```python
from build123d import *

# Parameters (mm, degrees)
SKETCH1_W                = 100
SKETCH1_H                = 110
BOSS_EXTRUDE1_DEPTH      = 6.86
BOSS_EXTRUDE2_DEPTH      = 6.86
CUT_EXTRUDE1_DEPTH       = 84.419927529
CUT_EXTRUDE1_DEPTH_BACK  = 84.419927529
CUT_EXTRUDE5_DEPTH       = 84.419927529
CUT_EXTRUDE6_DEPTH       = 84.419927529
SKETCH7_W                = 42
SKETCH7_H                = 3.55
CUT_EXTRUDE7_DEPTH       = 84.419927529
SKETCH8_W                = 5
SKETCH8_H                = 7.62
CUT_EXTRUDE8_DEPTH       = 84.419927529
CUT_EXTRUDE9_DEPTH       = 84.419927529
LPATTERN1_COUNT          = 2
LPATTERN1_PITCH          = 49.4
SKETCH15_W               = 6.5
SKETCH15_H               = 9.5
BOSS_EXTRUDE3_DEPTH      = 6.86
CUT_EXTRUDE14_START      = -6.86
CUT_EXTRUDE14_DEPTH      = 6.86
BOSS_EXTRUDE4_DEPTH      = 6.86
FILLET3_R                = 5
FILLET4_R                = 7
CUT_EXTRUDE11_DEPTH      = 84.419927529
BOSS_EXTRUDE5_DEPTH      = 6.86
CUT_EXTRUDE12_DEPTH      = 84.419927529
CUT_EXTRUDE12_DEPTH_BACK = 84.419927529
SKETCH21_R               = 1
CUT_EXTRUDE13_DEPTH      = 84.419927529
CUT_EXTRUDE15_DEPTH      = 84.419927529
CUT_EXTRUDE15_DEPTH_BACK = 84.419927529
CUT_EXTRUDE16_DEPTH      = 84.419927529
CUT_EXTRUDE16_DEPTH_BACK = 84.419927529
FILLET2_R                = 1
BOSS_EXTRUDE6_DEPTH      = 6.86
CUT_EXTRUDE17_DEPTH      = 84.419927529
BOSS_EXTRUDE9_DEPTH      = 6.86


# Read off the part's stored shape, not the designer's step: Cut-Extrude14
with BuildPart() as part:
    # Sketch1 → Boss-Extrude1 (new body)
    with BuildSketch(Plane.XY):
        Rectangle(SKETCH1_W, SKETCH1_H)
    extrude(amount=BOSS_EXTRUDE1_DEPTH)

    # Sketch14 → Boss-Extrude2 (add)
    with BuildSketch(Plane.XY.offset(6.86)):
        with BuildLine():
            Line((-50, 44), (-56.9, 44))
            Line((-56.9, 44), (-57.252653961, 46))
            Line((-57.252653961, 46), (-60.252653961, 46))
            ThreePointArc((-60.252653961, 46), (-62.140394827, 27.177051725), (-56.9, 9))
            Line((-56.9, 9), (-50, 9))
            Line((-50, 9), (-50, 44))
        make_face()
    extrude(amount=-BOSS_EXTRUDE2_DEPTH)

    # Sketch9 → Cut-Extrude1 (cut, two sides: drawn at the far end of the back side and taken through both)
    with BuildSketch(Plane.XY.offset(6.86).offset(-CUT_EXTRUDE1_DEPTH_BACK)):
        Polygon((-202.691345573, 326.397371639), (-46, 55), (2.5, -29.004464167), (-49.825975731, -59.214880341), (-321.22334737, -215.906225914), (291.08659924, -349.739606366), (409.618601037, 192.563991188), align=None)
    extrude(amount=CUT_EXTRUDE1_DEPTH + CUT_EXTRUDE1_DEPTH_BACK, mode=Mode.SUBTRACT)

    # Sketch11 → Cut-Extrude5 (cut, through all)
    with BuildSketch(Plane.XY.offset(6.86)):
        Polygon((-35.90593882, 37.516573181), (-8.20593882, -10.461234188), (-15.13414205, -14.461234188), (-42.83414205, 33.516573181), align=None)
    extrude(amount=-CUT_EXTRUDE5_DEPTH, mode=Mode.SUBTRACT)

    # Sketch12 → Cut-Extrude6 (cut, through all)
    with BuildSketch(Plane.XY.offset(6.86)):
        Polygon((-18.88414205, -7.96604366), (-21.534179786, -9.49604366), (-35.534179786, 14.752667646), (-32.88414205, 16.282667646), align=None)
    extrude(amount=-CUT_EXTRUDE6_DEPTH, mode=Mode.SUBTRACT)

    # Sketch7 → Cut-Extrude7 (cut, through all)
    with BuildSketch(Plane.XY.offset(6.86)):
        with Locations((-50, -34)):
            Rectangle(SKETCH7_W, SKETCH7_H)
    extrude(amount=-CUT_EXTRUDE7_DEPTH, mode=Mode.SUBTRACT)

    # Sketch8 → Cut-Extrude8 (cut, through all)
    with BuildSketch(Plane.XY.offset(6.86)):
        with Locations((-36.5, -34)):
            Rectangle(SKETCH8_W, SKETCH8_H)
    extrude(amount=-CUT_EXTRUDE8_DEPTH, mode=Mode.SUBTRACT)

    # Sketch13 → Cut-Extrude9 (cut, through all)
    with BuildSketch(Plane.XY.offset(6.86)):
        Polygon((-41.88414205, 31.871124914), (-40.78414205, 29.965869026), (-48.578370684, 25.465869026), (-48.078370684, 24.599843622), (-49.508178626, 23.774343622), (-50.008178626, 24.640369026), (-52.908497703, 22.965869026), (-54.008497703, 24.871124914), (-51.108178626, 26.545624914), (-51.608178626, 27.411650318), (-50.178370684, 28.237150318), (-49.678370684, 27.371124914), align=None)
        Polygon((-39.45593882, 43.665353548), (-38.35593882, 41.76009766), (-46.150167454, 37.26009766), (-45.650167454, 36.394072256), (-47.079975396, 35.568572256), (-47.579975396, 36.43459766), (-50.480294473, 34.76009766), (-51.580294473, 36.665353548), (-48.679975396, 38.339853548), (-49.179975396, 39.205878952), (-47.750167454, 40.031378952), (-47.250167454, 39.165353548), align=None)
        Polygon((-18.443009001, -24.930108514), (-11.443009001, -37.054464167), (-9.537753113, -35.954464167), (-16.537753113, -23.830108514), align=None)
    cut_extrude9 = extrude(amount=-CUT_EXTRUDE9_DEPTH, mode=Mode.SUBTRACT)

    # LPattern1: Cut-Extrude9 ×2
    with Locations(*[Vector(0.4999999999999939, -0.8660254037844421, 0) * (i * LPATTERN1_PITCH) for i in range(1, LPATTERN1_COUNT)]):
        add(cut_extrude9, mode=Mode.SUBTRACT)

    # Sketch15 → Boss-Extrude3 (add)
    with BuildSketch(Plane.XY.offset(6.86)):
        with Locations((-53.25, -19.75)):
            Rectangle(SKETCH15_W, SKETCH15_H)
    extrude(amount=-BOSS_EXTRUDE3_DEPTH)

    # Cut-Extrude14 outline → Cut-Extrude14 (cut)
    with BuildSketch(Plane.XY.offset(6.86).offset(CUT_EXTRUDE14_START)):
        Polygon((-56.5, -15), (-56.5, -16.500643242), (-50, -15), align=None)
    extrude(amount=CUT_EXTRUDE14_DEPTH, mode=Mode.SUBTRACT)

    # Sketch16 → Boss-Extrude4 (add)
    with BuildSketch(Plane.XY.offset(6.86)):
        Polygon((-35.605117767, -51.004464167), (-34.105117767, -53.602540378), (-36.525588833, -55), (-42.525588833, -55), (-44.558274136, -51.479285778), align=None)
    extrude(amount=-BOSS_EXTRUDE4_DEPTH)

    # Fillet3
    fillet3_edges = [part.edges().sort_by_distance(p)[0] for p in [
        (2.5, -29.004464167, 3.43),
    ]]
    fillet(fillet3_edges, radius=FILLET3_R)

    # Fillet4
    fillet4_edges = [part.edges().sort_by_distance(p)[0] for p in [
        (-56.9, 9, 3.43),
    ]]
    fillet(fillet4_edges, radius=FILLET4_R)

    # Sketch18 → Cut-Extrude11 (cut, through all)
    with BuildSketch(Plane.XY.offset(6.86)):
        Polygon((-17.634534405, -28.330427591), (-13.997227709, -26.230427591), (-13.171727709, -27.660235533), (-16.809034405, -29.760235533), align=None)
    extrude(amount=-CUT_EXTRUDE11_DEPTH, mode=Mode.SUBTRACT)

    # Sketch19 → Boss-Extrude5 (add)
    with BuildSketch(Plane.XY.offset(6.86)):
        Polygon((-24.334179786, -4.646301399), (-23.234179786, -6.551557287), (-25.780294473, -8.021557287), (-26.880294473, -6.116301399), align=None)
    extrude(amount=-BOSS_EXTRUDE5_DEPTH)

    # Sketch20 → Cut-Extrude12 (cut, two sides: drawn at the far end of the back side and taken through both)
    with BuildSketch(Plane.XY.offset(6.86).offset(-CUT_EXTRUDE12_DEPTH_BACK)):
        Polygon((-50, 55), (-50, 44), (-48.060403212, 55), align=None)
    extrude(amount=CUT_EXTRUDE12_DEPTH + CUT_EXTRUDE12_DEPTH_BACK, mode=Mode.SUBTRACT)

    # Sketch21 → Cut-Extrude13 (cut, through all)
    with BuildSketch(Plane.XY.offset(6.86)):
        with Locations((-38, -5)):
            Circle(SKETCH21_R)
    extrude(amount=-CUT_EXTRUDE13_DEPTH, mode=Mode.SUBTRACT)

    # Sketch23 → Cut-Extrude15 (cut, two sides: drawn at the far end of the back side and taken through both)
    with BuildSketch(Plane.XY.offset(6.86).offset(-CUT_EXTRUDE15_DEPTH_BACK)):
        Polygon((207.425051562, 16.452548282), (-35.605117767, -51.004464167), (-50, -55), (-293.030169328, -122.457012449), (-158.11614443, -608.517351106), (342.33907646, -469.607790375), align=None)
    extrude(amount=CUT_EXTRUDE15_DEPTH + CUT_EXTRUDE15_DEPTH_BACK, mode=Mode.SUBTRACT)

    # Sketch25 → Cut-Extrude16 (cut, two sides: drawn at the far end of the back side and taken through both)
    with BuildSketch(Plane(origin=(0, 0, 0), x_dir=(-1, 0, 0), z_dir=(0, 0, -1)).offset(-CUT_EXTRUDE16_DEPTH_BACK)):
        Polygon((-209.546353054, 0.01089), (35.605117767, -51.004464167), (50, -54), (295.15147082, -105.015354167), (193.120762486, -595.318295807), (-311.577061387, -490.29205164), align=None)
    extrude(amount=CUT_EXTRUDE16_DEPTH + CUT_EXTRUDE16_DEPTH_BACK, mode=Mode.SUBTRACT)

    # Fillet2
    fillet2_edges = [part.edges().sort_by_distance(p)[0] for p in [
        (-60.252653961, 46, 3.43),
        (-56.5, -24.5, 3.43),
        (-56.5, -16.500643242, 3.43),
        (-50, -54, 3.43),
    ]]
    fillet(fillet2_edges, radius=FILLET2_R)

    # Sketch26 → Boss-Extrude6 (add)
    with BuildSketch(Plane(origin=(0, 0, 0), x_dir=(-1, 0, 0), z_dir=(0, 0, -1))):
        with BuildLine():
            Line((56.5, -15), (50, -15))
            Line((50, -15), (55.724951054, -16.321709094))
            ThreePointArc((55.724951054, -16.321709094), (56.282608157, -16.673564522), (56.5, -17.296079159))
            Line((56.5, -17.296079159), (56.5, -15))
        make_face()
        Polygon((47.579975396, 36.43459766), (50, 35.037395803), (50, 37.577736987), (48.679975396, 38.339853548), (49.179975396, 39.205878952), (47.750167454, 40.031378952), (47.250167454, 39.165353548), (39.45593882, 43.665353548), (38.35593882, 41.76009766), (46.150167454, 37.26009766), (45.650167454, 36.394072256), (47.079975396, 35.568572256), align=None)
        Polygon((49.678370684, 27.371124914), (41.88414205, 31.871124914), (40.78414205, 29.965869026), (48.578370684, 25.465869026), (48.078370684, 24.599843622), (49.508178626, 23.774343622), (50, 24.62620323), (50, 27.92820323), align=None)
        with BuildLine():
            ThreePointArc((56.5, -23.5), (56.207106781, -24.207106781), (55.5, -24.5))
            Line((55.5, -24.5), (56.5, -24.5))
            Line((56.5, -24.5), (56.5, -23.5))
        make_face()
    extrude(amount=-BOSS_EXTRUDE6_DEPTH)

    # Sketch26<3> → Cut-Extrude17 (cut, through all)
    with BuildSketch(Plane(origin=(0, 0, 0), x_dir=(-1, 0, 0), z_dir=(0, 0, -1))):
        with BuildLine():
            Line((50, 35.037395803), (50, 27.92820323))
            Line((50, 27.92820323), (50.178370684, 28.237150318))
            Line((50.178370684, 28.237150318), (51.608178626, 27.411650318))
            Line((51.608178626, 27.411650318), (51.108178626, 26.545624914))
            Line((51.108178626, 26.545624914), (54.008497703, 24.871124914))
            Line((54.008497703, 24.871124914), (52.908497703, 22.965869026))
            Line((52.908497703, 22.965869026), (50.008178626, 24.640369026))
            Line((50.008178626, 24.640369026), (50, 24.62620323))
            Line((50, 24.62620323), (50, 9))
            Line((50, 9), (52.380008746, 9))
            ThreePointArc((52.380008746, 9), (56.324728806, 10.217337668), (58.897432775, 13.445947531))
            ThreePointArc((58.897432775, 13.445947531), (62.283923616, 29.230647449), (60.464218102, 45.271649399))
            ThreePointArc((60.464218102, 45.271649399), (60.105291207, 45.797386167), (59.50182182, 46))
            Line((59.50182182, 46), (57.252653961, 46))
            Line((57.252653961, 46), (56.9, 44))
            Line((56.9, 44), (50, 44))
            Line((50, 44), (50, 37.577736987))
            Line((50, 37.577736987), (51.580294473, 36.665353548))
            Line((51.580294473, 36.665353548), (50.480294473, 34.76009766))
            Line((50.480294473, 34.76009766), (50, 35.037395803))
        make_face()
        with BuildLine():
            Line((55.724951054, -16.321709094), (50, -15))
            Line((50, -15), (50, -24.5))
            Line((50, -24.5), (55.5, -24.5))
            ThreePointArc((55.5, -24.5), (56.207106781, -24.207106781), (56.5, -23.5))
            Line((56.5, -23.5), (56.5, -17.296079159))
            ThreePointArc((56.5, -17.296079159), (56.282608157, -16.673564522), (55.724951054, -16.321709094))
        make_face()
        with BuildLine():
            Line((56.5, -15), (50, -15))
            Line((50, -15), (55.724951054, -16.321709094))
            ThreePointArc((55.724951054, -16.321709094), (56.282608157, -16.673564522), (56.5, -17.296079159))
            Line((56.5, -17.296079159), (56.5, -15))
        make_face()
        with BuildLine():
            ThreePointArc((56.5, -23.5), (56.207106781, -24.207106781), (55.5, -24.5))
            Line((55.5, -24.5), (56.5, -24.5))
            Line((56.5, -24.5), (56.5, -23.5))
        make_face()
    extrude(amount=-CUT_EXTRUDE17_DEPTH, mode=Mode.SUBTRACT)

    # Sketch29 → Boss-Extrude9 (add)
    with BuildSketch(Plane(origin=(0, 0, 0), x_dir=(-1, 0, 0), z_dir=(0, 0, -1))):
        Polygon((39, -35.775), (50, -35.775), (50, -32.225), (39, -32.225), (39, -30.19), (34, -30.19), (34, -32.225), (29, -32.225), (29, -35.775), (34, -35.775), (34, -37.81), (39, -37.81), align=None)
        Polygon((50, 44), (50, 55), (48.060403212, 55), align=None)
    extrude(amount=-BOSS_EXTRUDE9_DEPTH)


solid = part.part
```
Could you check a few things on this model? Use its own coordinates, in mm. A direction names the side the tool comes from. Round coordinates to 2 decimals unless told otherwise and drop trailing zeros. Loops run counter-clockwise (first coordinate to the right, second up) from the corner with the lowest first, then second, coordinate; pieces in that order, holes last. Notation, with made-up numbers: M -23.75,-14.75 L -10.75,-14.75 A16 ccw -10.75,-8.75 Z; hole C -25.75,58 d7. An arc over 180 degrees is marked long. Answer as CSV lines item,"result".
1) Imagine slicing it at A-A on x = -4. List the corners of the cut face in (y, z) for me.
From the geometry:
outline,"M -32.76,0 L -17.75,0 L -17.75,6.86 L -32.76,6.86 Z"
2) For pin 1 Ø3 at (x, z) = (-26, 2.5) entering from -Y (3 decimals); pin 2 Ø4 at (x, z) = (-32.5, 1) entering from +Y; pin 3 Ø1.5 at (x, z) = (-31, 1) entering from -Y, each with a flat end and sliding along its axis, tell me the tip position at first contact or that it passes through.
From the geometry:
pin 1,"y = -46.325"
pin 2,"y = 19.08"
pin 3,"y = -48.78"
3) Imagine slicing it at B-B on y = 13. List the corners of the cut face in (x, z) for me.
From the geometry:
outline,"M -50,0 L -34.52,0 L -34.52,6.86 L -50,6.86 Z"
4) Which directions (+Z, -Z, +X, -X, +Y, -Y) give clear straight access to the entire face, cutting with the end or side of a thin tool? Please do faces 5 (the flat face through (-20.19, -8.72, 3.48)), 6 (the flat face through (-5.63, -33.7, 3.38)), 7 (the flat face through (-34.228, 15.507, 3.478)), 8 (the flat face through (-17.617, -26.36, 3.478)).
From the geometry:
face 5,"+Z, -Z, +Y"
face 6,"+Z, -Z, +X, -Y"
face 7,"+Z, -Z, +X"
face 8,"+Z, -Z"
5) If I drill on probe 1 along Y at (x, z) = (-38, 3.5); probe 2 along Y at (x, z) = (-18, 2); probe 3 along X at (y, z) = (2, 6), over which ranges is the centre line in solid material (lowest first)?
From the geometry:
probe 1,"-51.5 to -6, -4 to 25.14, 36.31 to 41.14"
probe 2,"-40.84 to -25.7, -24.67 to -13.92, -11.38 to -9.5"
probe 3,"-50 to -28.17"
6) We'd pull the mould along Y, two halves only. Please class faces 1 (the flat face through (-21.136, -13.192, 3.478)), 2 (the flat face through (-48, 55, 3)), 3 (the flat face through (-36, -11, 0)), 4 (the cylindrical face through (-37, -5, 3)): released by +Y, released by -Y, zero draft, split by the parting line, or undercut.
From the geometry:
face 1,"undercut"
face 2,"released by +Y"
face 3,"zero draft"
face 4,"undercut"
